Input: part model. Units: mm. Frame: model coordinates. A direction names the side the tool comes from. Give positions to 0.01 mm unless a question says otherwise; leave off trailing zeros. Write each loop counter-clockwise with the first axis right and the second up, starting at its lowest first coordinate (ties: lowest second). Pieces come first, ordered by that corner, then holes. Notation, with made-up numbers: (69, -31.5) -> (111, -31.5) arc R23 ccw to (111, 7.5) -> close; hole circle Ø7 at (49, 28.25). An arc over 180 degrees is marked (long way). Return JSON: item names as keys, results as strings. Group by question number.
Item 1: Section A-A, the plane y = 0. Return loops of the section in (x, z), then the cut area to 3 significant figures.
Item 2: Line query: line 1 (Z direction, x = -18, y = -1.5); line 2 (X direction, y = -0.75, z = -4); line 3 (X direction, y = -1.5, z = 3.25). Output: solid intervals per line, ascending. Write a range as [from, to].
Item 3: Set-up query: faces 1 (the face through (50.365, -0.088, 1.972)), 2 (the face through (-31.727, 0.601, 5.972)), 3 (the face through (44.458, 0.601, -3.944)). Return all of +Z, -Z, +X, -X, +Y, -Y with unobstructed straight access to the full face (end or side cutting, diameter ignored); none if empty.
Item 4: Section C-C, the plane z = 1.5. Return loops of the section in (x, y).
Item 5: Pin query (flat end, axial travel): P1, Ø1, axis at x = -20.5, y = 0, coming from the -Z side; P2, Ø2.5, axis at x = 25, y = 1, coming from the +Z side; P3, Ø3, axis at y = 2, z = 4.5, coming from the -X side. Return the tip coordinate at first contact, or that it passes through.
Item 6: Section B-B, the plane x = 14. Return loops of the section in (y, z), then the cut area to 3 significant figures.
from build123d import *

# Parameters (mm, degrees)
EXTRUDE_1_DEPTH = 4
SKETCH_2_R      = 2
EXTRUDE_2_DEPTH = 8
SKETCH_3_R      = 2
EXTRUDE_3_DEPTH = 4


with BuildPart() as part:
    # 草图1 → 凸台-拉伸1 (new body)
    with BuildSketch(Plane.XY):
        with BuildLine():
            Line((-33.634370857, -4), (46.365629143, -4))
            ThreePointArc((46.365629143, -4), (50.365629143, 0), (46.365629143, 4))
            Line((46.365629143, 4), (-33.634370857, 4))
            ThreePointArc((-33.634370857, 4), (-37.634370857, 0), (-33.634370857, -4))
        make_face()
    extrude(amount=EXTRUDE_1_DEPTH)

    # 草图2 → 凸台-拉伸2 (add)
    with BuildSketch(Plane(origin=(0, 0, 0), x_dir=(-1, 0, 0), z_dir=(0, 0, -1))):
        with Locations((-46.365629143, 0)):
            Circle(SKETCH_2_R)
    extrude(amount=EXTRUDE_2_DEPTH)

    # 草图3 → 凸台-拉伸3 (add)
    with BuildSketch(Plane.XY.offset(4)):
        with Locations((-33.634370857, 0)):
            Circle(SKETCH_3_R)
    extrude(amount=EXTRUDE_3_DEPTH)


solid = part.part
Answer below:
{
 "1": {"outline": "(-37.63, 0) -> (44.37, 0) -> (44.37, -8) -> (48.37, -8) -> (48.37, 0) -> (50.37, 0) -> (50.37, 4) -> (-31.63, 4) -> (-31.63, 8) -> (-35.63, 8) -> (-35.63, 4) -> (-37.63, 4) -> close", "area": "400 mm2"},
 "2": {"line 1": "z = [0, 4]", "line 2": "x = [44.51, 48.22]", "line 3": "x = [-37.34, 50.07]"},
 "3": {"face 1": "+Z, -Z, +X", "face 2": "+Z", "face 3": "-Z"},
 "4": {"outline": "(-33.63, -4) -> (46.37, -4) arc R4 ccw to (46.37, 4) -> (-33.63, 4) arc R4 ccw to start"},
 "5": {"P1": "stops at z = 0", "P2": "stops at z = 4", "P3": "stops at x = -37.59"},
 "6": {"outline": "(-4, 0) -> (4, 0) -> (4, 4) -> (-4, 4) -> close", "area": "32.0 mm2"}
}
